Check sheet for the modelled part. Datum: model origin and axes. Units: mm. A direction names the side the tool comes from. Round coordinates to 2 decimals unless told otherwise and drop trailing zeros. Order: outer loops, then holes, each group sorted by start corner. A loop starts at its lowest first (then second) coordinate and runs counter-clockwise, first axis right, second up.
```python
from build123d import *

# Parameters (mm, degrees)
F0_W     = 24.64179
F0_H     = 25.4
F1_DEPTH = 25.4
F2_R     = 3.8735
F2_R_2   = 3.87346
F3_DEPTH = 22.86


with BuildPart() as f1:
    # F0 (on Front) → F1 (new body)
    with BuildSketch(Plane.XZ):
        Rectangle(F0_W, F0_H)
    extrude(amount=F1_DEPTH)

    # F2 (on face) → F3 (cut)
    with BuildSketch(Plane.XZ.offset(25.4)):
        Polygon((8.611645, -4.853836), (-8.611646, -4.853836), (-4.540686, -8.298493), (0, -8.298493), (5.793288, -8.298493), align=None)
        with Locations((4.540684, 6.106439)):
            Circle(F2_R)
        with Locations((-7.359042, 6.106439)):
            Circle(F2_R_2)
    extrude(amount=-F3_DEPTH, mode=Mode.SUBTRACT)


solid = f1.part
```
Item 1: Sectioned sample at C-C (z = 6.5). Record the cut outline in (x, y), and give its area (3 significant figures).
Answer:
outline: (-12.32, -25.4) - (-11.21, -25.4) - (-11.21, -2.54) - (-3.51, -2.54) - (-3.51, -25.4) - (0.69, -25.4) - (0.69, -2.54) - (8.39, -2.54) - (8.39, -25.4) - (12.32, -25.4) - (12.32, 0) - (-12.32, 0) - close
area: 274 mm2
Item 2: Sectioned sample at D-D (x = 3). Record the cut outline in (y, z).
Answer:
outline: (-25.4, -12.7) - (0, -12.7) - (0, 12.7) - (-25.4, 12.7) - (-25.4, 9.66) - (-2.54, 9.66) - (-2.54, 2.55) - (-25.4, 2.55) - (-25.4, -4.85) - (-2.54, -4.85) - (-2.54, -8.3) - (-25.4, -8.3) - close
Item 3: Sectioned sample at B-B (x = -2.75). Record the cut outline in (y, z), and give its area (3 significant figures).
Answer:
outline: (-25.4, -12.7) - (0, -12.7) - (0, 12.7) - (-25.4, 12.7) - (-25.4, -4.85) - (-2.54, -4.85) - (-2.54, -8.3) - (-25.4, -8.3) - close
area: 566 mm2
Item 4: Go/stop test with a flat-tipped pin: P1, Ø1.7, axis at x = 3.5, z = -6, coming from the -Y side. Record where the tip stops, or that it passes through.
Answer:
P1: stops at y = -2.54
Item 5: Access from +Z, -Z, +X, -X, +Y, -Y to the whole of each face (thin tool, end or side, straight path). Record for faces 1 (the flat face through (0, 0, 0)), 2 (the flat face through (0, -2.54, -7)).
Answer:
face 1: +Z, -Z, +X, -X, +Y
face 2: -Y
Item 6: Sectioned sample at A-A (y = -5). Record the cut outline in (x, z), and give its area (3 significant figures).
Answer:
outline: (-12.32, -12.7) - (12.32, -12.7) - (12.32, 12.7) - (-12.32, 12.7) - close; hole circle Ø7.75 at (-7.36, 6.11); hole (-8.61, -4.85) - (-4.54, -8.3) - (5.79, -8.3) - (8.61, -4.85) - close; hole circle Ø7.75 at (4.54, 6.11)
area: 484 mm2
Item 7: Scan lines: line 1 along Z through (x, y) = (4.5, -10); line 2 along Z through (x, y) = (-0.75, -23.5); line 3 along Z through (x, y) = (7.25, -19.5). Record each from-to range of solid material in increasing order.
Answer:
line 1: z = -12.7 to -8.3, -4.85 to 2.23, 9.98 to 12.7
line 2: z = -12.7 to -8.3, -4.85 to 12.7
line 3: z = -12.7 to -6.52, -4.85 to 3.34, 8.87 to 12.7
Item 8: Release check for a two-part mould opening along X. For faces 3 (the flat face through (12.321, -13, 0)), 4 (the flat face through (0, -25.4, 0)), 5 (the flat face through (-7, -2.54, 6)) record: released by +X, released by -X, zero draft, split by the parting line, or undercut.
Answer:
face 3: released by +X
face 4: zero draft
face 5: undercut
